Source: CAD feature listing. Evaluate the final solid. Frame: model axes, mm. A direction names the side the tool comes from. Give positions to 0.01 mm unless a question says otherwise; leave off trailing zeros. Order: outer loops, then holes, each group sorted by start corner. A loop starts at its lowest first (then second) coordinate and runs counter-clockwise, first axis right, second up. Notation, with made-up numbers: (-36, -23) - (-5, -23) arc R20 cw to (-5, -18) - close; hole circle Ø11 at (78.25, 33). An arc over 180 degrees is marked (long way). Answer as CSV lines item,"result".
```python
from build123d import *

# Parameters (mm, degrees)
SKETCH3_R           = 5
SKETCH3_R_2         = 0.8
BOSS_EXTRUDE1_DEPTH = 4


with BuildPart() as part:
    # Sketch2 → luer (revolve)
    with BuildSketch(Plane.XY, mode=Mode.PRIVATE) as luer_sk:
        with BuildLine():
            Line((-1.05, 0), (-2.213, 0))
            Line((-2.213, 0), (-1.785190896, 8.163083989))
            ThreePointArc((-1.785190896, 8.163083989), (-1.707622156, 8.331343593), (-1.535533512, 8.4))
            Line((-1.535533512, 8.4), (-1.05, 8.4))
            Line((-1.05, 8.4), (-1.05, 0))
        make_face()
    revolve(luer_sk.sketch.rotate(Axis((0, 0, 0), (0, 1, 0)), 270), axis=Axis((0, 0, 0), (0, 1, 0)))

    # Sketch3 → Boss-Extrude1 (add)
    with BuildSketch(Plane.XZ):
        with Locations(Location((0, 0, 0), (0, 0, 270))):
            Circle(SKETCH3_R)
        with Locations(Location((0, 0, 0), (0, 0, 270))):
            Circle(SKETCH3_R_2, mode=Mode.SUBTRACT)
    extrude(amount=BOSS_EXTRUDE1_DEPTH)


solid = part.part
```
(1) Cut plane D-D (z = 4). Return loops of the section in (x, y), then the cut area to 3 significant figures.
Completed:
outline,"(-3, -4) - (3, -4) - (3, 0) - (-3, 0) - close"
area,"24.0 mm²"
(2) Mould query, pull axis Z, two halves, no side actions, for faces 1 (the conical face through (-1.98, 4.14, 0.26)), 2 (the cylindrical face through (-0.32, 4.14, -1)), 3 (the flat face through (1, 8.4, -0.7)). Classes: released by +Z, released by -Z, zero draft, split by the parting line, or undercut.
Completed:
face 1,"split by the parting line"
face 2,"undercut"
face 3,"zero draft"
(3) Cut plane A-A (z = 0). Return loops of the section in (x, y).
Completed:
outline,"(-5, -4) - (-0.8, -4) - (-0.8, 0) - (-1.05, 0) - (-1.05, 8.4) - (-1.54, 8.4) arc R0.25 ccw to (-1.79, 8.16) - (-2.21, 0) - (-5, 0) - close; (0.8, -4) - (5, -4) - (5, 0) - (2.21, 0) - (1.79, 8.16) arc R0.25 ccw to (1.54, 8.4) - (1.05, 8.4) - (1.05, 0) - (0.8, 0) - close"
(4) Contact query for flat-ended pins moving along their axis: pin 1 (2 mm diameter, centred on y = 7, z = -2.5, fed in from +X); pin 2 (2 mm diameter, centred on y = 7, z = 4, fed in from -X); pin 3 (2.5 mm diameter, centred on x = 0, z = 0, fed in from +Y); pin 4 (1 mm diameter, centred on y = -1.5, z = 1, fed in from -X). Output: stop coordinate, or through.
Completed:
pin 1,"x = 1.08"
pin 2,"through"
pin 3,"y = 8.4"
pin 4,"x = -4.97"
(5) Cut plane C-C (y = 2). Return loops of the section in (x, z).
Completed:
outline,"circle Ø4.22 at (0, 0); hole circle Ø2.1 at (0, 0)"
(6) Cut plane B-B (x = 0). Return loops of the section in (y, z).
Completed:
outline,"(-4, -5) - (0, -5) - (0, -2.21) - (8.16, -1.79) arc R0.25 ccw to (8.4, -1.54) - (8.4, -1.05) - (0, -1.05) - (0, -0.8) - (-4, -0.8) - close; (-4, 0.8) - (0, 0.8) - (0, 1.05) - (8.4, 1.05) - (8.4, 1.54) arc R0.25 ccw to (8.16, 1.79) - (0, 2.21) - (0, 5) - (-4, 5) - close"
(7) Access query for faces 4 (the flat face through (-1, 0, -2.2)), 5 (the cylindrical face through (-4.88, -1.97, 1.08)). Directions: +Z, -Z, +X, -X, +Y, -Y. A direction counts if a zero-diameter tool reaches every point of the face in a straight line with its end or side. Return the directions, or none.
Completed:
face 4,"+Y"
face 5,"+Y, -Y"
(8) Ray query, line 1 (X direction, y = -2.75, z = 0); line 2 (X direction, y = 6.75, z = 0); line 3 (Y direction, x = -3, z = -1). Return the intervals inside material, ascending. Write a range as from..to.
Completed:
line 1,"-5..-0.8, 0.8..5"
line 2,"-1.86..-1.05, 1.05..1.86"
line 3,"-4..0"
